```python
from build123d import *

# Parameters (mm, degrees)
SKETCH1_R           = 1
BOSS_EXTRUDE1_DEPTH = 6.5
SKETCH2_R           = 1.25
BOSS_EXTRUDE2_DEPTH = 0.5
BOSS_EXTRUDE3_START = 0.5
SKETCH3_R           = 1.25
BOSS_EXTRUDE3_DEPTH = 0.5
SKETCH4_R           = 0.75
CUT_EXTRUDE1_DEPTH  = 10.5
FILLET1_R           = 0.25


with BuildPart() as part:
    # Sketch1 → Boss-Extrude1 (new body)
    with BuildSketch(Plane.XY):
        with Locations(Location((0, 0, 0), (0, 0, 180))):
            Circle(SKETCH1_R)
    extrude(amount=BOSS_EXTRUDE1_DEPTH)

    # Sketch2 → Boss-Extrude2 (add)
    with BuildSketch(Plane.XY.offset(6.5)):
        Circle(SKETCH2_R)
    extrude(amount=BOSS_EXTRUDE2_DEPTH)

    # Sketch3 → Boss-Extrude3 (add)
    with BuildSketch(Plane(origin=(0, 0, 0), x_dir=(-1, 0, 0), z_dir=(0, 0, -1)).offset(BOSS_EXTRUDE3_START)):
        with Locations(Location((0, 0, 0), (0, 0, 180))):
            Circle(SKETCH3_R)
    extrude(amount=-BOSS_EXTRUDE3_DEPTH)

    # Sketch4 → Cut-Extrude1 (cut)
    with BuildSketch(Plane.XY.offset(7)):
        Circle(SKETCH4_R)
    extrude(amount=-CUT_EXTRUDE1_DEPTH, mode=Mode.SUBTRACT)

    # Fillet1
    fillet1_edges = [part.edges().sort_by_distance(p)[0] for p in [
        (-1.25, 0, -0.5),
        (-0.75, 0, -0.5),
        (-0.75, 0, 7),
        (-1.25, 0, 7),
    ]]
    fillet(fillet1_edges, radius=FILLET1_R - 0.0001)  # a hair under: the kernel refuses the full size


solid = part.part
```
The listing builds one solid part. Answer for the finished solid, in the listing's coordinates (mm). Give positions to 0.01 mm unless a question says otherwise; leave off trailing zeros. Loops run counter-clockwise (first coordinate to the right, second up) from the corner with the lowest first, then second, coordinate; pieces in that order, holes last. Notation, with made-up numbers: (-13, 57.5) - (11, 57.5) arc R15 cw to (11, 76.5) - close; hole circle Ø7 at (57, 56). An arc over 180 degrees is marked (long way). Return JSON: item names as keys, results as strings. Group by question number.
1. Determine the mould class of faces 1 (the cylindrical face through (-0.75, 0.03, 3.3)), 2 (the cylindrical face through (0, 1, 3)) for opening direction Z: pulls with the +Z half, pulls with the -Z half, needs draft (parallel to the pull), parting line crosses it, or undercut.
2. Find section B-B (z = 1.5). Write down the section's boundary in (x, y), then the cut area to 3 significant figures.
3. Straight lines are drawn through the part: line 1 (Y direction, x = 0, z = 1.5); line 2 (Y direction, x = 0.4, z = 1); line 3 (X direction, y = 0.45, z = 1). For each, find the intervals that lie inside material, in ascending order. Write a range as [from, to].
4. Given pin 1 Ø1 at (x, z) = (0.5, 1.5) entering from -Y, flat-ended and moving along its own axis, determine where the tip first touches the part or whether it passes through.
Verdict:
{
 "1": {"face 1": "needs draft", "face 2": "undercut"},
 "2": {"outline": "circle Ø2 at (0, 0); hole circle Ø1.5 at (0, 0)", "area": "1.37 mm^2"},
 "3": {"line 1": "y = [-1, -0.75], [0.75, 1]", "line 2": "y = [-0.92, -0.63], [0.63, 0.92]", "line 3": "x = [-0.89, -0.6], [0.6, 0.89]"},
 "4": {"pin 1": "stops at y = -1"}
}
